Check sheet for the modelled part. Datum: model origin and axes. Units: mm. Give positions to 0.01 mm unless a question says otherwise; leave off trailing zeros. Order: outer loops, then holes, each group sorted by start corner. A loop starts at its lowest first (then second) coordinate and runs counter-clockwise, first axis right, second up.
Item 1: Gauge pin test, flat end, axial feed: P1, Ø24, axis at x = 70.73, z = 14, coming from the -Y side (3 decimals). Record the tip position at first contact, or that the pin passes through.
Item 2: Sectioned sample at B-B on x = -4.5. Record the boundary of the cut face in (y, z), and give its area (3 significant figures).
Item 3: Sectioned sample at A-A on z = 20. Record the boundary of the cut face in (x, y).
Item 4: Material ranges on line 1 along Z through (x, y) = (-8.5, -3); line 2 along Z through (x, y) = (64, -1.5); line 3 along X through (y, z) = (-3.75, 27.5), recorded low to high.
from build123d import *

# Parameters (mm, degrees)
F0_W     = 500
F0_H     = 220
F0_R     = 15
F0_R_2   = 14.456537
F1_DEPTH = 12


with BuildPart() as f1:
    # F0 (on Front) → F1 (new body)
    with BuildSketch(Plane.XZ):
        with Locations((5.457865, -9.454479)):
            Rectangle(F0_W, F0_H)
        with Locations((-4.772537, -40)):
            Circle(F0_R, mode=Mode.SUBTRACT)
        with Locations((-90.26964, -17.208472)):
            Circle(F0_R, mode=Mode.SUBTRACT)
        with Locations((67.227463, -26)):
            Circle(F0_R, mode=Mode.SUBTRACT)
        with Locations((31.227463, -20)):
            Circle(F0_R_2, mode=Mode.SUBTRACT)
        with Locations((2.227463, 0)):
            Circle(F0_R, mode=Mode.SUBTRACT)
        with Locations((70.727463, 14)):
            Circle(F0_R, mode=Mode.SUBTRACT)
        with Locations((35.227463, 20)):
            Circle(F0_R, mode=Mode.SUBTRACT)
    extrude(amount=F1_DEPTH)


solid = f1.part
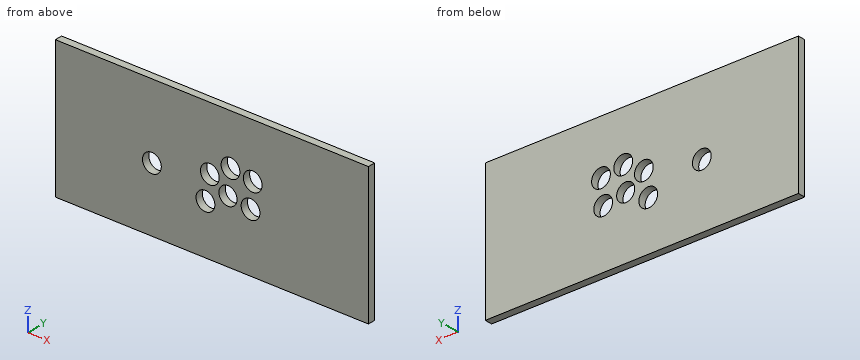
Report:
1. P1: passes through
2. outline: (-12, -119.45) - (0, -119.45) - (0, -55) - (-12, -55) - close; (-12, -25) - (0, -25) - (0, -13.41) - (-12, -13.41) - close; (-12, 13.41) - (0, 13.41) - (0, 100.55) - (-12, 100.55) - close
2. area: 1,960 mm2
3. outline: (-244.54, -12) - (20.23, -12) - (20.23, 0) - (-244.54, 0) - close; (50.23, -12) - (56.98, -12) - (56.98, 0) - (50.23, 0) - close; (84.48, -12) - (255.46, -12) - (255.46, 0) - (84.48, 0) - close
4. line 1: z = -119.45 to -54.53, -25.47 to -10.48, 10.48 to 100.55
4. line 2: z = -119.45 to -40.65, -11.35 to 0.59, 27.41 to 100.55
4. line 3: x = -244.54 to 22.24, 48.22 to 64.19, 77.27 to 255.46
